```python
from build123d import *

# Parameters (mm, degrees)
F0_R           = 25
F1_DEPTH       = 30
F3_DEPTH       = 4
F4_R           = 15
F5_DEPTH       = 14
F6_W           = 13
F6_H           = 13
F7_DEPTH       = 30.001
F8_R           = 25
F8_R_2         = 15
F9_DEPTH       = 13
F10_R          = 3
F11_DEPTH      = 25.001
F11_DEPTH_BACK = 25.001
F12_S5_R       = 3
F12_T6_DEPTH   = 32
F13_R          = 0.15
F14_R          = 2


# Not quite as in the source:
# - a fillet or chamfer that OpenCascade refuses, or shapes differently, is made with other operations: its cross-section is extruded or revolved along the edge and cut away or added


with BuildPart() as f1:
    # F0 (on Top) → F1 (new body)
    with BuildSketch(Plane.XY):
        Circle(F0_R)
    extrude(amount=F1_DEPTH)

    # F2 (on face) → F3 (cut)
    with BuildSketch(Plane.XY.offset(30)):
        with BuildLine():
            Line((16.7009618943, 11.1423048454), (1.2990381057, 20.0346096908))
            ThreePointArc((1.2990381057, 20.0346096908), (0, 19.2846096908), (-1.2990381057, 20.0346096908))
            Line((-1.2990381057, 20.0346096908), (-16.7009618943, 11.1423048454))
            ThreePointArc((-16.7009618943, 11.1423048454), (-16.5511112606, 10.7805334131), (-16.5, 10.3923048454))
            ThreePointArc((-16.5, 10.3923048454), (-16.9393398282, 9.3316446736), (-18, 8.8923048454))
            Line((-18, 8.8923048454), (-18, -8.8923048454))
            ThreePointArc((-18, -8.8923048454), (-16.9393398282, -9.3316446736), (-16.5, -10.3923048454))
            ThreePointArc((-16.5, -10.3923048454), (-16.5511112606, -10.7805334131), (-16.7009618943, -11.1423048454))
            Line((-16.7009618943, -11.1423048454), (-1.2990381057, -20.0346096908))
            ThreePointArc((-1.2990381057, -20.0346096908), (0, -19.2846096908), (1.2990381057, -20.0346096908))
            Line((1.2990381057, -20.0346096908), (16.7009618943, -11.1423048454))
            ThreePointArc((16.7009618943, -11.1423048454), (16.7009618943, -9.6423048454), (18, -8.8923048454))
            Line((18, -8.8923048454), (18, 8.8923048454))
            ThreePointArc((18, 8.8923048454), (16.7009618943, 9.6423048454), (16.7009618943, 11.1423048454))
        make_face()
        with BuildLine():
            ThreePointArc((-16.5, 10.3923048454), (-16.5511112606, 10.7805334131), (-16.7009618943, 11.1423048454))
            Line((-16.7009618943, 11.1423048454), (-18, 10.3923048454))
            Line((-18, 10.3923048454), (-18, 8.8923048454))
            ThreePointArc((-18, 8.8923048454), (-16.9393398282, 9.3316446736), (-16.5, 10.3923048454))
        make_face()
        with BuildLine():
            ThreePointArc((-16.5, -10.3923048454), (-16.9393398282, -9.3316446736), (-18, -8.8923048454))
            Line((-18, -8.8923048454), (-18, -10.3923048454))
            Line((-18, -10.3923048454), (-16.7009618943, -11.1423048454))
            ThreePointArc((-16.7009618943, -11.1423048454), (-16.5511112606, -10.7805334131), (-16.5, -10.3923048454))
        make_face()
        with BuildLine():
            Line((0, -20.7846096908), (1.2990381057, -20.0346096908))
            ThreePointArc((1.2990381057, -20.0346096908), (0, -19.2846096908), (-1.2990381057, -20.0346096908))
            Line((-1.2990381057, -20.0346096908), (0, -20.7846096908))
        make_face()
        with BuildLine():
            Line((18, -10.3923048454), (18, -8.8923048454))
            ThreePointArc((18, -8.8923048454), (16.7009618943, -9.6423048454), (16.7009618943, -11.1423048454))
            Line((16.7009618943, -11.1423048454), (18, -10.3923048454))
        make_face()
        with BuildLine():
            Line((18, 10.3923048454), (16.7009618943, 11.1423048454))
            ThreePointArc((16.7009618943, 11.1423048454), (16.7009618943, 9.6423048454), (18, 8.8923048454))
            Line((18, 8.8923048454), (18, 10.3923048454))
        make_face()
        with BuildLine():
            Line((1.2990381057, 20.0346096908), (0, 20.7846096908))
            Line((0, 20.7846096908), (-1.2990381057, 20.0346096908))
            ThreePointArc((-1.2990381057, 20.0346096908), (0, 19.2846096908), (1.2990381057, 20.0346096908))
        make_face()
    extrude(amount=-F3_DEPTH, mode=Mode.SUBTRACT)

    # F4 (on face) → F5 (cut)
    with BuildSketch(Plane.XY.offset(30)):
        Circle(F4_R)
    extrude(amount=-F5_DEPTH, mode=Mode.SUBTRACT)

    # F6 (on face) → F7 (cut, through all)
    with BuildSketch(Plane(origin=(0, 0, 0), x_dir=(1, 0, 0), z_dir=(0, 0, -1))):
        Rectangle(F6_W, F6_H)
    extrude(amount=-F7_DEPTH, mode=Mode.SUBTRACT)

    # F8 (on face) → F9 (cut)
    with BuildSketch(Plane(origin=(0, 0, 0), x_dir=(1, 0, 0), z_dir=(0, 0, -1))):
        Circle(F8_R)
        Circle(F8_R_2, mode=Mode.SUBTRACT)
    extrude(amount=-F9_DEPTH, mode=Mode.SUBTRACT)

    # F10 (on Front) → F11 (cut, two sides)
    with BuildSketch(Plane.XZ) as f11_sk:
        with Locations((0, 8)):
            Circle(F10_R)
    extrude(amount=-F11_DEPTH, mode=Mode.SUBTRACT)
    extrude(f11_sk.sketch, amount=F11_DEPTH_BACK, mode=Mode.SUBTRACT)

    # F12: fillet of radius 5 on 1 edges, made by hand


with BuildPart() as f12_tool2:
    # F12_s3 → F12_t4 (revolve)
    with BuildSketch(Plane.XZ):
        with BuildLine():
            ThreePointArc((20, 13), (16.4644660941, 11.5355339059), (15, 8))
            Line((15, 8), (15, 13))
            Line((15, 13), (20, 13))
        make_face()
    revolve(axis=Axis((0, 0, 13), (0, 0, -1)))

    # F12_s5 → F12_t6 (cut, symmetric)
    with BuildSketch(Plane.XZ):
        with Locations((0, 8)):
            Circle(F12_S5_R)
    extrude(amount=F12_T6_DEPTH, both=True, mode=Mode.SUBTRACT)


with BuildPart() as f1_1:
    add(f1.part)

    # F12_t1: union F12_tool2
    add(f12_tool2.part)

    # F13
    f13_edges = [f1_1.edges().sort_by_distance(p)[0] for p in [
        (-6.5, -6.5, 8),
        (-6.5, 6.5, 8),
        (6.5, 6.5, 8),
        (6.5, -6.5, 8),
    ]]
    fillet(f13_edges, radius=F13_R)

    # F14
    f14_edges = [f1_1.edges().sort_by_distance(p)[0] for p in [
        (-18, -10.392305, 28),
        (-18, 10.392305, 28),
        (0, -20.78461, 28),
        (18, -10.392305, 28),
        (18, 10.392305, 28),
        (0, 20.78461, 28),
    ]]
    fillet(f14_edges, radius=F14_R)


solid = f1_1.part
```
Source: CAD feature listing. Evaluate the final solid. Frame: model axes, mm. A direction names the side the tool comes from. Round coordinates to 2 decimals unless told otherwise and drop trailing zeros. Loops run counter-clockwise (first coordinate to the right, second up) from the corner with the lowest first, then second, coordinate; pieces in that order, holes last.
(1) Section query B-B (x = 0). Output: boundary loops of the cut face in (y, z), and give its area (3 significant figures).
From the geometry:
outline: (-25, 13) - (-20, 13) arc R5 cw to (-16, 11) - (-6.5, 11) - (-6.5, 16) - (-15, 16) - (-15, 26) - (-20.48, 26) - (-20.48, 30) - (-25, 30) - close; (-15, 0) - (-6.5, 0) - (-6.5, 5) - (-15, 5) - close; (6.5, 0) - (15, 0) - (15, 5) - (6.5, 5) - close; (6.5, 11) - (16, 11) arc R5 cw to (20, 13) - (25, 13) - (25, 30) - (20.48, 30) - (20.48, 26) - (15, 26) - (15, 16) - (6.5, 16) - close
area: 475 mm2
(2) Contact query for flat-ended pins moving along their axis: pin 1 Ø2 at (x, y) = (-14.5, -5.5) entering from +Z; pin 2 Ø3 at (x, y) = (-1, -12) entering from +Z; pin 3 Ø2 at (x, z) = (-2, 14.5) entering from -Y; pin 4 Ø10 at (x, y) = (-7.5, -10.5) entering from -Z. Output: stop coordinate, or through.
From the geometry:
pin 1: stops at z = 26
pin 2: stops at z = 16
pin 3: stops at y = -24.98
pin 4: stops at z = 0
(3) Section query D-D (z = 24). Output: boundary loops of the cut face in (x, y), and give its area (3 significant figures).
From the geometry:
outline: circle Ø50 at (0, 0); hole circle Ø30 at (0, 0)
area: 1,260 mm2
(4) Access query for faces 4 (the cylindrical face through (17.725, 10.25, 27.972)), 5 (the cylindrical face through (-3.252, 14.643, 3.944)), 6 (the flat face through (3, 6.5, 6)). Directions: +Z, -Z, +X, -X, +Y, -Y. A direction counts if a zero-diameter tool reaches every point of the face in a straight line with its end or side. Return the directions, or none.
From the geometry:
face 4: +Z
face 5: -Z
face 6: +Z, -Z
(5) Section query A-A (y = 0). Output: boundary loops of the cut face in (x, z).
From the geometry:
outline: (-25, 13) - (-20, 13) arc R5 cw to (-15, 8) - (-15, 0) - (-6.5, 0) - (-6.5, 16) - (-15, 16) - (-15, 26) - (-18, 26) - (-18, 30) - (-25, 30) - close; (6.5, 0) - (15, 0) - (15, 8) arc R5 cw to (20, 13) - (25, 13) - (25, 30) - (18, 30) - (18, 26) - (15, 26) - (15, 16) - (6.5, 16) - close
(6) Pull-direction query (Z, two-part tool) for faces 1 (the flat face through (0, 7, 0)), 2 (the cylindrical face through (-17.725, 10.25, 27.972)), 3 (the flat face through (0, 7, 16)); classes: +Z half, -Z half, draft (parallel to the pull), parting line (faces both ways), or undercut.
From the geometry:
face 1: -Z half
face 2: draft
face 3: +Z half
(7) Material intervals for probe 1 along Z at (x, y) = (0, -10); probe 2 along X at (y, z) = (2.5, 3.5); probe 3 along Z at (x, y) = (14, 2), sorted ascending.
From the geometry:
probe 1: z = 0 to 5, 11 to 16
probe 2: x = -14.79 to -6.5, 6.5 to 14.79
probe 3: z = 0 to 16
(8) Section query C-C (z = 27.5). Output: boundary loops of the cut face in (x, y).
From the geometry:
outline: circle Ø50 at (0, 0); hole (-18, -9.24) arc R2 ccw to (-17, -10.97) - (-1, -20.21) arc R2 ccw to (1, -20.21) - (17, -10.97) arc R2 ccw to (18, -9.24) - (18, 9.24) arc R2 ccw to (17, 10.97) - (1, 20.21) arc R2 ccw to (-1, 20.21) - (-17, 10.97) arc R2 ccw to (-18, 9.24) - close
